Autodesk Inventor part; units mm, degrees
ref_plane "YZ Plane" through (0, 0, 0) normal (1, 0, 0) x (0, 1, 0)
ref_plane "XZ Plane" through (0, 0, 0) normal (0, 1, 0) x (-1, 0, 0)
ref_plane "XY Plane" through (0, 0, 0) normal (0, 0, 1) x (1, 0, 0)
sketch "Sketch1" plane through (0, 0, 0) normal (0, 0, 1) x (1, 0, 0)
  circle A0 centre (0, 0) radius 9.5
  dimension "d0" = 19
extrude "Extrusion1" add sketch "Sketch1" along normal blind 3
sketch "Sketch2" plane through (0, 0, 3) normal (0, 0, 1) x (1, 0, 0)
  circle A0 centre (0, 0) radius 9.5
  circle A1 centre (0, 0) radius 4
  dimension "d3" = 8
extrude "Extrusion2" add sketch "Sketch2" along normal blind 2 contours A1
sketch "Sketch3" plane through (0, 0, 5) normal (0, 0, 1) x (1, 0, 0)
  circle A0 centre (0, 0) radius 4
  circle A1 centre (0, 0) radius 2.5
  dimension "d6" = 5
extrude "Extrusion3" add sketch "Sketch3" along normal blind 1 contours A1
fillet "Fillet1" radius 1 1 edges at (-2.5, 0, 6)
sketch "Sketch4" plane through (0, 0, 3) normal (0, 0, 1) x (1, 0, 0)
  circle A0 centre (0, 0) radius 4
  line L0 (0, 4) -> (0, 9.5)
  circle A1 centre (0, 0) radius 9.5
  line L1 (-9.5, 0) -> (-4, 0)
  line L2 (-13.3, 0) -> (13.3, 0) construction
  line L3 (0, -13.3) -> (0, 13.3) construction
  circle A2 centre (0, 6.75) radius 1.5
  circle A3 centre (0, -6.75) radius 1.5
  circle A4 centre (-6.75, 0) radius 1.5
  circle A5 centre (6.75, 0) radius 1.5
  dimension "d10" = 3
extrude "Extrusion4" cut sketch "Sketch4" against normal through all contours A2 L0 | L0 A2 | A4 L1 | L1 A4 | A3 | A5
sketch "Sketch5" plane through (0, 0, 0) normal (0, 0, -1) x (-1, 0, 0)
  circle A0 centre (0, 0) radius 2.5
extrude "Extrusion5" add sketch "Sketch5" along normal blind 1
properties part number "FeeTechSTS3025BL-Flange"
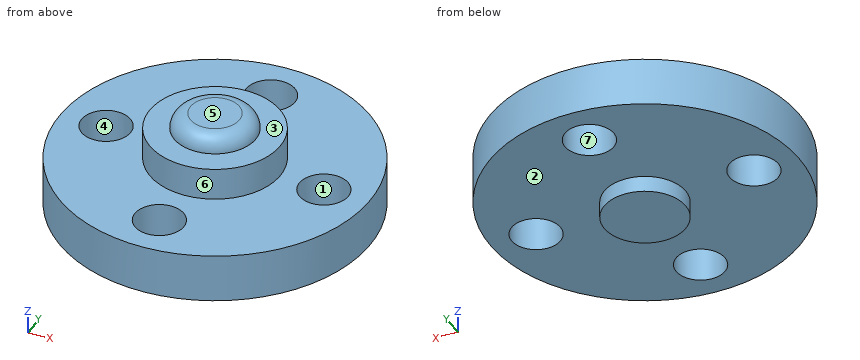
The listing builds one solid part. Answer for the finished solid, in the listing's coordinates (mm). Face numbers are marked on the shaded views. A direction names the side the tool comes from. Give positions to 0.01 mm unless a question says otherwise; leave off trailing zeros. Order: outer loops, then holes, each group sorted by start corner. A loop starts at its lowest first (then second) coordinate and runs counter-clockwise, first axis right, second up. Notation, with made-up numbers: (47.5, 64) - (95.5, 64) arc R29 ccw to (95.5, 88) - close; hole circle Ø7 at (41.5, -7.75). An arc over 180 degrees is marked (long way). Use one line per item in the form item = value. Start each with the question number.
(1) A cutting plane is placed at A-A, the plane x = 0. State how many separate pieces and enclosed holes the cut face has, then the cut area to 3 significant figures.
(2) A cutting plane is placed at C-C, the plane z = 2.5. Write down the section's boundary in (x, y).
(3) Consider line 1 (Y direction, x = 0, z = 0.85); line 2 (X direction, y = 1.25, z = 0.75); line 3 (Z direction, x = -4.5, y = -2.5). Determine where each line is inside the solid, lowest interval first. Write a range as from..to.
(4) The mould has two halves that part along X. Classify the marked faces 4, 5, 6 and 7: released by +X, released by -X, zero draft, split by the parting line, or undercut.
(5) For the marked faces 1, 2 and 3, determine the directions among +Z, -Z, +X, -X, +Y, -Y from which every point of the face is accessible in a straight line to the end or side of a thin tool.
(6) Flat-ended cylindrical pins translate along their axes: pin 1 Ø4 at (x, y) = (-1, -2) entering from +Z; pin 2 Ø4 at (x, y) = (0, -6.75) entering from -Z; pin 3 Ø4 at (y, z) = (4, 2) entering from -X; pin 4 Ø1 at (x, y) = (1.5, -7) entering from +Z. Find the tip coordinate at first contact, or state that the pin passes through.
(7) A cutting plane is placed at D-D, the plane y = 6.75. Write down the section's boundary in (x, z).
Ans:
q1.separate_pieces = 3
q1.enclosed_holes = 0
q1.area = 64.6 mm^2
q2.outline = circle Ø19 at (0, 0); hole circle Ø3 at (-6.75, 0); hole circle Ø3 at (0, -6.75); hole circle Ø3 at (0, 6.75); hole circle Ø3 at (6.75, 0)
q3.line_1 = -9.5..-8.25, -5.25..5.25, 8.25..9.5
q3.line_2 = -9.42..-7.58, -5.92..5.92, 7.58..9.42
q3.line_3 = 0..3
q4.face_4 = undercut
q4.face_5 = zero draft
q4.face_6 = split by the parting line
q4.face_7 = undercut
q5.face_1 = +Z, -Z
q5.face_2 = -Z
q5.face_3 = +Z
q6.pin_1 = 6
q6.pin_2 = 0
q6.pin_3 = -9.29
q6.pin_4 = 3
q7.outline = (-6.68, 0) - (-1.5, 0) - (-1.5, 3) - (-6.68, 3) - close; (1.5, 0) - (6.68, 0) - (6.68, 3) - (1.5, 3) - close
